from build123d import *

# Parameters (mm, degrees)
SKETCH1_W           = 9
SKETCH1_H           = 7
BOSS_EXTRUDE1_DEPTH = 6
CUT_EXTRUDE1_DEPTH  = 7
SKETCH3_W           = 5
SKETCH3_H           = 4
CUT_EXTRUDE2_DEPTH  = 1
SKETCH4_W           = 1
SKETCH4_H           = 1
CUT_EXTRUDE3_DEPTH  = 5
SKETCH5_W           = 1
SKETCH5_H           = 1.5
CUT_EXTRUDE4_DEPTH  = 3
SKETCH6_W           = 4
SKETCH6_H           = 1
CUT_EXTRUDE5_DEPTH  = 2
SKETCH7_W           = 1
SKETCH7_H           = 1.127539311
BOSS_EXTRUDE2_DEPTH = 2


with BuildPart() as part:
    # Sketch1 → Boss-Extrude1 (new body)
    with BuildSketch(Plane(origin=(0, 0, 0), x_dir=(1, 0, 0), z_dir=(0, 1, 0))):
        with Locations((4.5, 3.5)):
            Rectangle(SKETCH1_W, SKETCH1_H)
    extrude(amount=BOSS_EXTRUDE1_DEPTH)

    # Sketch2 → Cut-Extrude1 (cut)
    with BuildSketch(Plane.ZY):
        Polygon((0, 0), (-1, 0), (-1, 1), (-3, 4), (-6, 4), (-6, 6), (0, 6), align=None)
    extrude(amount=-CUT_EXTRUDE1_DEPTH, mode=Mode.SUBTRACT)

    # Sketch3 → Cut-Extrude2 (cut)
    with BuildSketch(Plane.ZY):
        with Locations((-3.5, 2)):
            Rectangle(SKETCH3_W, SKETCH3_H)
    extrude(amount=-CUT_EXTRUDE2_DEPTH, mode=Mode.SUBTRACT)

    # Sketch4 → Cut-Extrude3 (cut)
    with BuildSketch(Plane.XY):
        with Locations((7.5, 5.5)):
            Rectangle(SKETCH4_W, SKETCH4_H)
    extrude(amount=-CUT_EXTRUDE3_DEPTH, mode=Mode.SUBTRACT)

    # Sketch5 → Cut-Extrude4 (cut)
    with BuildSketch(Plane.ZY.offset(-1)):
        with Locations((-1.5, 1.75)):
            Rectangle(SKETCH5_W, SKETCH5_H)
    extrude(amount=-CUT_EXTRUDE4_DEPTH, mode=Mode.SUBTRACT)

    # Sketch6 → Cut-Extrude5 (cut)
    with BuildSketch(Plane(origin=(0, 6, 0), x_dir=(1, 0, 0), z_dir=(0, 1, 0))):
        with Locations((5, 6.5)):
            Rectangle(SKETCH6_W, SKETCH6_H)
    extrude(amount=-CUT_EXTRUDE5_DEPTH, mode=Mode.SUBTRACT)

    # Sketch7 → Boss-Extrude2 (add)
    with BuildSketch(Plane(origin=(0, 4, 0), x_dir=(1, 0, 0), z_dir=(0, 1, 0))):
        with Locations((2.5, 5.436230345)):
            Rectangle(SKETCH7_W, SKETCH7_H)
    extrude(amount=BOSS_EXTRUDE2_DEPTH)


solid = part.part
For this review, take the finished solid that the model builds, in its own axes (mm). A direction names the side the tool comes from. Round coordinates to 2 decimals unless told otherwise and drop trailing zeros. Order: outer loops, then holes, each group sorted by start corner. A loop starts at its lowest first (then second) coordinate and runs counter-clockwise, first axis right, second up. Notation, with made-up numbers: (4.5, 87) -> (43.5, 87) arc R34 ccw to (43.5, 119) -> close; hole circle Ø6 at (-11.75, 4.5). An arc over 180 degrees is marked (long way). Write item = value, one per line. Start each with the question number.
1) Tool access review of faces 4 (the face through (3, 5, -6)), 5 (the face through (7.5, 5.5, -5)), 6 (the face through (4.6, 2.8, -2.2)), 7 (the face through (1, 2, -4)): name each direction out of +Z, -Z, +X, -X, +Y, -Y from which nothing blocks a thin tool from reaching the whole face with its end or side.
2) Take a section at C-C on x = 4.5. State the section outline as (y, z) points, plus the area to 3 significant figures.
3) Take a section at B-B on z = -4.25. State the section outline as (x, y) points, plus the area to 3 significant figures.
4) Take a section at A-A on y = 4.35. State the section outline as (x, z) points, plus the area to 3 significant figures.
5) The part is to be moulded in two halves that separate along X. For faces 1 (the face through (7, 3, -2)), 2 (the face through (2, 2, -2)), 3 (the face through (2, 5, -5.4)), say which applies: +X half, -X half, draft (parallel to the pull), parting line (faces both ways), or undercut.
6) To check wall thickness, follow line 1 (X direction, y = 4.7, z = -6.5); line 2 (X direction, y = 4.15, z = -5.5); line 3 (X direction, y = 5.2, z = -0.75). State the ranges of each line that lie inside material, in increasing order. Write a range as from..to.
7) Insertion check: pin 1 (1.1 mm diameter, centred on x = 4.5, y = 0.5, fed in from +Z); pin 2 (0.8 mm diameter, centred on y = 5.5, z = -2, fed in from -X); pin 3 (1.1 mm diameter, centred on x = 2, z = -1.5, fed in from +Y) (3 decimals). Each pin has a flat end and moves straight along its axis. Give the tip position at first contact, or say it passes through.
8) Take a section at D-D on y = 0.55. State the section outline as (x, z) points.
Verdict:
q1.face_4 = +Z, -Z, +Y
q1.face_5 = +Z, +Y
q1.face_6 = +Z, -X, +Y
q1.face_7 = +Z, -X, +Y, -Y
q2.outline = (0, -7) -> (4, -7) -> (4, -3) -> (1, -1) -> (0, -1) -> close
q2.area = 21.0 mm2
q3.outline = (1, 0) -> (9, 0) -> (9, 6) -> (8, 6) -> (8, 5) -> (7, 5) -> (7, 4) -> (1, 4) -> close
q3.area = 35.0 mm2
q4.outline = (0, -7) -> (3, -7) -> (3, -4.87) -> (2, -4.87) -> (2, -6) -> (0, -6) -> close; (7, -7) -> (9, -7) -> (9, 0) -> (7, 0) -> close
q4.area = 18.1 mm2
q5.face_1 = undercut
q5.face_2 = draft
q5.face_3 = -X half
q6.line_1 = 0..3, 7..9
q6.line_2 = 2..3, 7..9
q6.line_3 = 8..9
q7.pin_1 = -1
q7.pin_2 = 8
q7.pin_3 = 2.575
q8.outline = (0, -7) -> (9, -7) -> (9, 0) -> (7, 0) -> (7, -1) -> (1, -1) -> (1, -6) -> (0, -6) -> close
